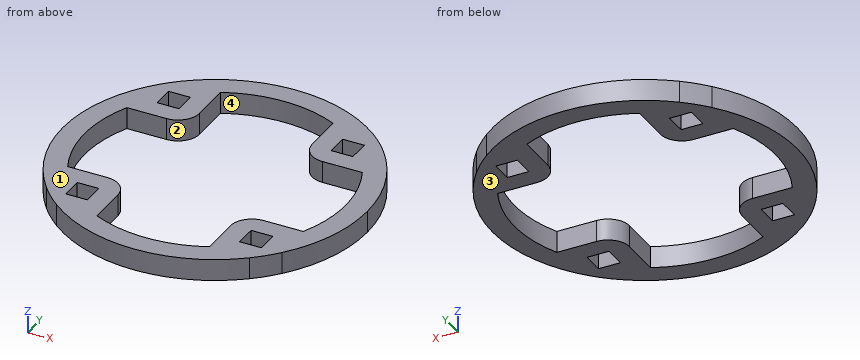
from build123d import *

# Parameters (mm, degrees)
F1_DEPTH = 10
F2_R     = 10


with BuildPart() as f1:
    # F0 (on Top) → F1 (new body)
    with BuildSketch(Plane.XY):
        with BuildLine():
            Line((-54.1421356237, 25.8578643763), (-54.1421356237, 44.3692365283))
            ThreePointArc((-54.1421356237, 44.3692365283), (-70, 0), (-54.1421356237, -44.3692365283))
            Line((-54.1421356237, -44.3692365283), (-54.1421356237, -25.8578643763))
            ThreePointArc((-54.1421356237, -25.8578643763), (-60, 0), (-54.1421356237, 25.8578643763))
        make_face()
        with BuildLine():
            Line((-25.8578643763, 54.1421356237), (-44.3692365283, 54.1421356237))
            ThreePointArc((-44.3692365283, 54.1421356237), (-49.4974746831, 49.4974746831), (-54.1421356237, 44.3692365283))
            Line((-54.1421356237, 44.3692365283), (-54.1421356237, 25.8578643763))
            ThreePointArc((-54.1421356237, 25.8578643763), (-50.0509436697, 33.0893190891), (-45, 39.686269666))
            Line((-45, 39.686269666), (-45, 45))
            Line((-45, 45), (-39.686269666, 45))
            ThreePointArc((-39.686269666, 45), (-33.0893190891, 50.0509436697), (-25.8578643763, 54.1421356237))
        make_face()
        with BuildLine():
            Line((25.8578643763, 54.1421356237), (44.3692365283, 54.1421356237))
            ThreePointArc((44.3692365283, 54.1421356237), (0, 70), (-44.3692365283, 54.1421356237))
            Line((-44.3692365283, 54.1421356237), (-25.8578643763, 54.1421356237))
            ThreePointArc((-25.8578643763, 54.1421356237), (0, 60), (25.8578643763, 54.1421356237))
        make_face()
        with BuildLine():
            Line((54.1421356237, 25.8578643763), (54.1421356237, 44.3692365283))
            ThreePointArc((54.1421356237, 44.3692365283), (49.4974746831, 49.4974746831), (44.3692365283, 54.1421356237))
            Line((44.3692365283, 54.1421356237), (25.8578643763, 54.1421356237))
            ThreePointArc((25.8578643763, 54.1421356237), (33.0893190891, 50.0509436697), (39.686269666, 45))
            Line((39.686269666, 45), (45, 45))
            Line((45, 45), (45, 39.686269666))
            ThreePointArc((45, 39.686269666), (50.0509436697, 33.0893190891), (54.1421356237, 25.8578643763))
        make_face()
        with BuildLine():
            ThreePointArc((54.1421356237, -44.3692365283), (65.9164224365, -23.5589739414), (70, 0))
            ThreePointArc((70, 0), (65.9164224365, 23.5589739414), (54.1421356237, 44.3692365283))
            Line((54.1421356237, 44.3692365283), (54.1421356237, 25.8578643763))
            ThreePointArc((54.1421356237, 25.8578643763), (58.5172117305, 13.2565429614), (60, 0))
            ThreePointArc((60, 0), (58.5172117305, -13.2565429614), (54.1421356237, -25.8578643763))
            Line((54.1421356237, -25.8578643763), (54.1421356237, -44.3692365283))
        make_face()
        with BuildLine():
            ThreePointArc((44.3692365283, -54.1421356237), (49.4974746831, -49.4974746831), (54.1421356237, -44.3692365283))
            Line((54.1421356237, -44.3692365283), (54.1421356237, -25.8578643763))
            ThreePointArc((54.1421356237, -25.8578643763), (50.0509436697, -33.0893190891), (45, -39.686269666))
            Line((45, -39.686269666), (45, -45))
            Line((45, -45), (39.686269666, -45))
            ThreePointArc((39.686269666, -45), (33.0893190891, -50.0509436697), (25.8578643763, -54.1421356237))
            Line((25.8578643763, -54.1421356237), (44.3692365283, -54.1421356237))
        make_face()
        with BuildLine():
            ThreePointArc((-44.3692365283, -54.1421356237), (0, -70), (44.3692365283, -54.1421356237))
            Line((44.3692365283, -54.1421356237), (25.8578643763, -54.1421356237))
            ThreePointArc((25.8578643763, -54.1421356237), (0, -60), (-25.8578643763, -54.1421356237))
            Line((-25.8578643763, -54.1421356237), (-44.3692365283, -54.1421356237))
        make_face()
        with BuildLine():
            ThreePointArc((-54.1421356237, -44.3692365283), (-49.4974746831, -49.4974746831), (-44.3692365283, -54.1421356237))
            Line((-44.3692365283, -54.1421356237), (-25.8578643763, -54.1421356237))
            ThreePointArc((-25.8578643763, -54.1421356237), (-33.0893190891, -50.0509436697), (-39.686269666, -45))
            Line((-39.686269666, -45), (-45, -45))
            Line((-45, -45), (-45, -39.686269666))
            ThreePointArc((-45, -39.686269666), (-50.0509436697, -33.0893190891), (-54.1421356237, -25.8578643763))
            Line((-54.1421356237, -25.8578643763), (-54.1421356237, -44.3692365283))
        make_face()
        Polygon((-35, -40), (-25.8578643763, -40), (-25.8578643763, -25.8578643763), (-40, -25.8578643763), (-40, -35), (-35, -35), align=None)
        with BuildLine():
            Line((-40, -25.8578643763), (-54.1421356237, -25.8578643763))
            ThreePointArc((-54.1421356237, -25.8578643763), (-50.0509436697, -33.0893190891), (-45, -39.686269666))
            Line((-45, -39.686269666), (-45, -35))
            Line((-45, -35), (-40, -35))
            Line((-40, -35), (-40, -25.8578643763))
        make_face()
        with BuildLine():
            ThreePointArc((-39.686269666, -45), (-33.0893190891, -50.0509436697), (-25.8578643763, -54.1421356237))
            Line((-25.8578643763, -54.1421356237), (-25.8578643763, -40))
            Line((-25.8578643763, -40), (-35, -40))
            Line((-35, -40), (-35, -45))
            Line((-35, -45), (-39.686269666, -45))
        make_face()
        with BuildLine():
            Line((25.8578643763, -40), (25.8578643763, -54.1421356237))
            ThreePointArc((25.8578643763, -54.1421356237), (33.0893190891, -50.0509436697), (39.686269666, -45))
            Line((39.686269666, -45), (35, -45))
            Line((35, -45), (35, -40))
            Line((35, -40), (25.8578643763, -40))
        make_face()
        Polygon((40, -35), (40, -25.8578643763), (25.8578643763, -25.8578643763), (25.8578643763, -40), (35, -40), (35, -35), align=None)
        with BuildLine():
            ThreePointArc((45, -39.686269666), (50.0509436697, -33.0893190891), (54.1421356237, -25.8578643763))
            Line((54.1421356237, -25.8578643763), (40, -25.8578643763))
            Line((40, -25.8578643763), (40, -35))
            Line((40, -35), (45, -35))
            Line((45, -35), (45, -39.686269666))
        make_face()
        with BuildLine():
            Line((40, 25.8578643763), (54.1421356237, 25.8578643763))
            ThreePointArc((54.1421356237, 25.8578643763), (50.0509436697, 33.0893190891), (45, 39.686269666))
            Line((45, 39.686269666), (45, 35))
            Line((45, 35), (40, 35))
            Line((40, 35), (40, 25.8578643763))
        make_face()
        Polygon((25.8578643763, 25.8578643763), (40, 25.8578643763), (40, 35), (35, 35), (35, 40), (25.8578643763, 40), align=None)
        with BuildLine():
            ThreePointArc((39.686269666, 45), (33.0893190891, 50.0509436697), (25.8578643763, 54.1421356237))
            Line((25.8578643763, 54.1421356237), (25.8578643763, 40))
            Line((25.8578643763, 40), (35, 40))
            Line((35, 40), (35, 45))
            Line((35, 45), (39.686269666, 45))
        make_face()
        with BuildLine():
            Line((-25.8578643763, 40), (-25.8578643763, 54.1421356237))
            ThreePointArc((-25.8578643763, 54.1421356237), (-33.0893190891, 50.0509436697), (-39.686269666, 45))
            Line((-39.686269666, 45), (-35, 45))
            Line((-35, 45), (-35, 40))
            Line((-35, 40), (-25.8578643763, 40))
        make_face()
        Polygon((-25.8578643763, 25.8578643763), (-25.8578643763, 40), (-35, 40), (-35, 35), (-40, 35), (-40, 25.8578643763), align=None)
        with BuildLine():
            ThreePointArc((-45, 39.686269666), (-50.0509436697, 33.0893190891), (-54.1421356237, 25.8578643763))
            Line((-54.1421356237, 25.8578643763), (-40, 25.8578643763))
            Line((-40, 25.8578643763), (-40, 35))
            Line((-40, 35), (-45, 35))
            Line((-45, 35), (-45, 39.686269666))
        make_face()
    extrude(amount=F1_DEPTH)

    # F2
    f2_edges = [f1.edges().sort_by_distance(p)[0] for p in [
        (25.857864, 25.857864, 5),
        (25.857864, -25.857864, 5),
        (-25.857864, 25.857864, 5),
        (-25.857864, -25.857864, 5),
    ]]
    fillet(f2_edges, radius=F2_R)


solid = f1.part
Build history of the part. All positions in model axes, mm. Face numbers are marked on the shaded views. A direction names the side the tool comes from. Give positions to 0.01 mm unless a question says otherwise; leave off trailing zeros. Write each loop counter-clockwise with the first axis right and the second up, starting at its lowest first coordinate (ties: lowest second). Pieces come first, ordered by that corner, then holes. Notation, with made-up numbers: (87, -23) - (104, -23) arc R22 cw to (104, -3) - close; hole circle Ø6 at (-33.75, 47.25). An arc over 180 degrees is marked (long way). Use one line per item in the form item = value. Start each with the question number.
1. Two-plate mould, pull along X, no slides. Class the marked faces 1 and 2: released by +X, released by -X, zero draft, split by the parting line, or undercut.
2. 3-axis set-ups, long thin cutter, end or side, ignore diameter. For the marked faces 3 and 4: which of +Z, -Z, +X, -X, +Y, -Y reach the whole face in a straight line?
3. Band-saw the part on B-B on x = 33. Write the cut outline in (y, z), plus the area to 3 significant figures.
4. Band-saw the part on A-A on y = -7. Write the cut outline in (x, z), plus the area to 3 significant figures.
5. Band-saw the part on D-D on z = 6. Count the separate pieces of the cut face and the enclosed holes in it, plus the area to 3 significant figures.
6. Probe line 1 (Y direction, x = -38.5, z = 4.25); line 2 (Y direction, x = 9.5, z = 5.5); line 3 (Y direction, x = 18.5, z = 5.5). List the from-to ranges inside material, lowest first. Write a range as [from, to].
7. Band-saw the part on C-C on x = -41.5. Write the cut outline in (y, z).
8. Drop flat-ended pins along their axis: pin 1 Ø5 at (x, z) = (42.5, 6) entering from -Y; pin 2 Ø6 at (y, z) = (56, 8.5) entering from -X; pin 3 Ø1 at (x, z) = (12.5, 7.5) entering from +Y. Give the stop position or say it passes through.
Conclusion:
q1.face_1 = zero draft
q1.face_2 = undercut
q2.face_3 = -Z, +X, -X, +Y, -Y
q2.face_4 = +Z, -Z
q3.outline = (-61.73, 0) - (-26.27, 0) - (-26.27, 10) - (-61.73, 10) - close; (26.27, 0) - (61.73, 0) - (61.73, 10) - (26.27, 10) - close
q3.area = 709 mm²
q4.outline = (-69.65, 0) - (-59.59, 0) - (-59.59, 10) - (-69.65, 10) - close; (59.59, 0) - (69.65, 0) - (69.65, 10) - (59.59, 10) - close
q4.area = 201 mm²
q5.separate_pieces = 1
q5.enclosed_holes = 5
q5.area = 5,570 mm²
q6.line_1 = [-58.46, -45], [-35, -25.86], [25.86, 35], [45, 58.46]
q6.line_2 = [-69.35, -59.24], [59.24, 69.35]
q6.line_3 = [-67.51, -57.08], [57.08, 67.51]
q7.outline = (-56.37, 0) - (-45, 0) - (-45, 10) - (-56.37, 10) - close; (-35, 0) - (-25.86, 0) - (-25.86, 10) - (-35, 10) - close; (25.86, 0) - (35, 0) - (35, 10) - (25.86, 10) - close; (45, 0) - (56.37, 0) - (56.37, 10) - (45, 10) - close
q8.pin_1 = -57.45
q8.pin_2 = -45.73
q8.pin_3 = 68.96
